Design review of the part built by this model. Coordinates are the model's own, in mm. Face numbers are marked on the shaded views. Coordinates: 2 decimals unless noted, no trailing zeros. Loops run counter-clockwise (first coordinate to the right, second up) from the corner with the lowest first, then second, coordinate; pieces in that order, holes last. Notation, with made-up numbers: M 59,20 L 118,20 A19 cw 118,57 Z; hole C -39,66.25 d8. An arc over 180 degrees is marked long. Answer as a JSON object with one key per item and string values. Group by question number.
1. Consider section A-A (x = 0). State the section outline as (y, z) points.
2. To check wall thickness, follow probe 1 along Y at (x, z) = (-14, 36); probe 2 along X at (y, z) = (15, 36); probe 3 along Z at (x, y) = (-58, 26.5). State the ranges of each line that lie inside material, in increasing order.
3. Draft analysis for pull direction X (two halves, no side actions). For the marked faces 1, 2 and 3, state which applies: +X half, -X half, draft (parallel to the pull), parting line (faces both ways), or undercut.
4. Consider section B-B (y = 50). State the section outline as (x, z) points.
5. Insertion check: pin 1 (1 mm diameter, centred on x = 34.5, z = -50.5, fed in from +Y); pin 2 (2 mm diameter, centred on y = 9.5, z = -27.5, fed in from +X); pin 3 (2 mm diameter, centred on y = 50.5, z = 65.5, fed in from +X); pin 4 (4.5 mm diameter, centred on x = 13.82, z = 8.07, fed in from -Y). Each pin has a flat end and moves straight along its axis. Give the tip position at first contact, or say it passes through.
Autodesk Inventor part; units mm, degrees
ref_plane "YZ Plane" through (0, 0, 0) normal (1, 0, 0) x (0, 1, 0)
ref_plane "XZ Plane" through (0, 0, 0) normal (0, 1, 0) x (-1, 0, 0)
ref_plane "XY Plane" through (0, 0, 0) normal (0, 0, 1) x (1, 0, 0)
sketch "Эскиз2" plane through (0, 0, 0) normal (1, 0, 0) x (0, 1, 0)
  line L0 (0, 16.9979) -> (0, -102.0021)
  line L1 (18.2354, -0.0021) -> (-21.7975, -0.0021) construction
  line L2 (0, -85.0021) -> (4, -85.0021)
  line L3 (4, -85.0021) -> (4, -79.0021)
  line L4 (4, -75.0021) -> (65, -75.0021)
  line L5 (65, -75.0021) -> (65, -78.0021)
  line L6 (65, -79.0021) -> (65, -75.0021) construction
  line L7 (4, -79.0021) -> (55, -79.0021)
  line L8 (55, -79.0021) -> (65, -78.0021)
  line L9 (4, -75.0021) -> (4, -4.0021)
  line L10 (0, -85.0021) -> (0, -4.0021)
  line L11 (0, -4.0021) -> (4, -4.0021)
  point P0 (0, -0.0021)
  point P1 (4, -0.0021)
  dimension "d1" = 4
  dimension "d2" = 6
  dimension "d3" = 61
  dimension "d6" = 3
  dimension "d7" = 51
  dimension "d8" = 4
revolve "Вращение1" add sketch "Эскиз2" angle 360 about axis through (0, 18.2354, -0.0021) along (0, -1, 0)
fillet "Сопряжение1" radius 1 1 edges at (0, 4, 74.9979)
sketch "Эскиз3" plane through (0, 4, -0.0021) normal (0, 1, 0) x (1, 0, 0)
  ellipse E0 centre (-13.967, 8.3729) end of major axis (-13.9806, 5.1229) minor radius 3.25 construction
  circle A0 centre (13.8163, -8.069) radius 3.25 construction
  circle A1 centre (13.8163, -8.069) radius 2.5
  circle A2 centre (-13.967, 8.3729) radius 2.5
  arc A3 (-64.2334, 5.859) -> (-62.6955, 4.3359) centre (-65.4333, 3.1094) ccw
  circle A4 centre (-65.4333, 3.1094) radius 5
  point P0 (0, -0.0021)
  dimension "d14" = 10
extrude "Выдавливание1" cut sketch "Эскиз3" against normal blind 10
properties part number "Cap_pipes"
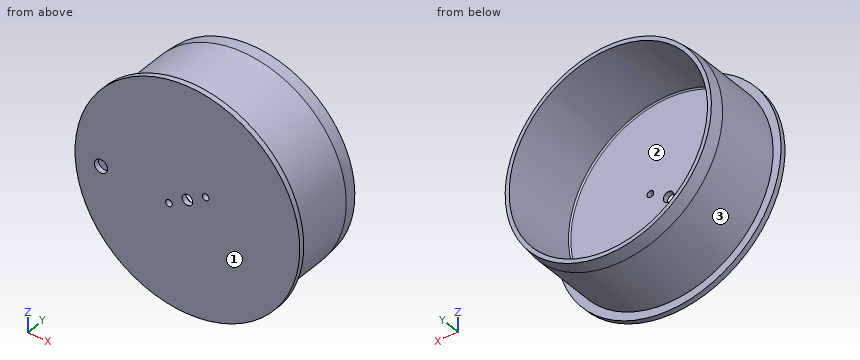
Findings below:
{
 "1": {"outline": "M 0,-85 L 4,-85 L 4,-79 L 55,-79 L 65,-78 L 65,-75 L 5,-75 A1 cw 4,-74 L 4,-4 L 0,-4 Z; M 0,4 L 4,4 L 4,74 A1 cw 5,75 L 65,75 L 65,78 L 55,79 L 4,79 L 4,85 L 0,85 Z"},
 "2": {"probe 1": "y = 0 to 4", "probe 2": "x = -70.32 to -65.79, 65.79 to 70.32", "probe 3": "z = -53.64 to -47.55, 47.55 to 53.64"},
 "3": {"face 1": "draft", "face 2": "undercut", "face 3": "parting line"},
 "4": {"outline": "C 0,0 d158; hole C 0,0 d150"},
 "5": {"pin 1": "stops at y = 4", "pin 2": "stops at x = 74.42", "pin 3": "stops at x = 45.61", "pin 4": "passes through"}
}
